Geometry check sheet. Reference: the model listing, model coordinates, mm. A direction names the side the tool comes from. Give positions to 0.01 mm unless a question says otherwise; leave off trailing zeros. Loops run counter-clockwise (first coordinate to the right, second up) from the corner with the lowest first, then second, coordinate; pieces in that order, holes last. Notation, with made-up numbers: (25.25, -20) - (58.25, -20) arc R16 ccw to (58.25, -16) - close; hole circle Ø7 at (-34.5, -17.5). An arc over 180 degrees is marked (long way). Write item = value, one per line. Start each with the question number.
from build123d import *

# Parameters (mm, degrees)
BOSS_EXTRUDE1_DEPTH = 2
SKETCH2_R           = 4
SKETCH2_R_2         = 3
BOSS_EXTRUDE2_DEPTH = 3.5
FILLET1_R           = 2.5
SKETCH3_R           = 1.5
CUT_EXTRUDE1_DEPTH  = 2


with BuildPart() as part:
    # Sketch1 → Boss-Extrude1 (new body)
    with BuildSketch(Plane(origin=(0, 0, 0), x_dir=(1, 0, 0), z_dir=(0, 1, 0))):
        with BuildLine():
            Line((-24.810790305, 12.959420841), (-17.699288905, 2.803144292))
            ThreePointArc((-17.699288905, 2.803144292), (-17.300062844, 1.904277974), (-17.699288905, 1.005411656))
            Line((-17.699288905, 1.005411656), (-24.810790305, -9.150864893))
            ThreePointArc((-24.810790305, -9.150864893), (-24.5530862, -12.096436293), (-21.6075148, -12.354140399))
            Line((-21.6075148, -12.354140399), (-11.45123825, -5.242638998))
            ThreePointArc((-11.45123825, -5.242638998), (-10.552371933, -4.843412937), (-9.653505615, -5.242638998))
            Line((-9.653505615, -5.242638998), (0.502770934, -12.354140399))
            ThreePointArc((0.502770934, -12.354140399), (3.448342335, -12.096436293), (3.70604644, -9.150864893))
            Line((3.70604644, -9.150864893), (-3.40545496, 1.005411656))
            ThreePointArc((-3.40545496, 1.005411656), (-3.804681022, 1.904277974), (-3.40545496, 2.803144292))
            Line((-3.40545496, 2.803144292), (3.70604644, 12.959420841))
            ThreePointArc((3.70604644, 12.959420841), (3.448342335, 15.904992242), (0.502770934, 16.162696347))
            Line((0.502770934, 16.162696347), (-9.653505615, 9.051194947))
            ThreePointArc((-9.653505615, 9.051194947), (-10.552371933, 8.651968885), (-11.45123825, 9.051194947))
            Line((-11.45123825, 9.051194947), (-21.6075148, 16.162696347))
            ThreePointArc((-21.6075148, 16.162696347), (-24.5530862, 15.904992242), (-24.810790305, 12.959420841))
        make_face()
    extrude(amount=BOSS_EXTRUDE1_DEPTH)

    # Sketch2 → Boss-Extrude2 (add)
    with BuildSketch(Plane.XZ):
        with Locations(Location((-10.552371933, -1.904277974, 0), (0, 0, 90))):
            Circle(SKETCH2_R)
        with Locations(Location((-10.552371933, -1.904277974, 0), (0, 0, 270))):
            Circle(SKETCH2_R_2, mode=Mode.SUBTRACT)
    extrude(amount=BOSS_EXTRUDE2_DEPTH)

    # Fillet1
    fillet1_edges = [part.edges().sort_by_distance(p)[0] for p in [
        (-10.552371933, 0, -5.904277974),
    ]]
    fillet(fillet1_edges, radius=FILLET1_R)

    # Sketch3 → Cut-Extrude1 (cut)
    with BuildSketch(Plane.XZ):
        with Locations(Location((-10.552371933, -1.904277974, 0), (0, 0, 270))):
            Circle(SKETCH3_R)
    extrude(amount=-CUT_EXTRUDE1_DEPTH, mode=Mode.SUBTRACT)


solid = part.part
1) Cross-section at C-C on y = 0.45. Enter the section's corners in (x, z).
2) Release check for a two-part mould opening along X. For faces 1 (the face through (-21.305, 0.986, -7.952)), 2 (the face through (-7.004, -2.993, -0.059)), 3 (the face through (0.1, 0.99, -7.81)), 4 (the face through (3.416, 0.986, 12.128)) record: pulls with the +X half, pulls with the -X half, needs draft (parallel to the pull), parting line crosses it, or undercut.
3) Cross-section at D-D on y = -1.6. Enter the section's corners in (x, z), and give its area (3 significant figures).
4) Material ranges on line 1 along Y through (x, z) = (-17.5, 0.5); line 2 along Z through (x, y) = (-22.5, 1.5); line 3 along Z through (x, y) = (-11.75, -0.9), recorded low to high.
5) Cross-section at A-A on x = -20.5. Enter the section's corners in (y, z), and give its area (3 significant figures).
6) Cross-section at B-B on z = -14.5. Enter the section's corners in (x, y), and give its area (3 significant figures).
7) Tool access check on faces 5 (the face through (-7.58, -1.73, -1.51)), 6 (the face through (0.2, 0.986, 4.144)), 7 (the face through (-16.6, 0.99, 8.85)), 8 (the face through (-21.205, 0.986, 4.002)), 9 (the face through (-16.46, 0.99, -12.56)). Record the directions out of +Z, -Z, +X, -X, +Y, -Y that give a thin tool (end or side, any length) a straight path to the whole face; none if there is none.
8) Gauge pin test, flat ends, axial feed: P1, Ø3, axis at y = 0, z = 6.5, coming from the -X side; P2, Ø5, axis at x = -10.55, z = -1.9, coming from the -Y side; P3, Ø1.5, axis at y = -3, z = -6, coming from the -X side. Record the tip position at first contact, or that the pin passes through.
Checked values:
q1.outline = (-24.81, -12.96) arc R2.3 ccw to (-21.61, -16.16) - (-11.45, -9.05) arc R1.21 cw to (-9.65, -9.05) - (0.5, -16.16) arc R2.3 ccw to (3.71, -12.96) - (-3.41, -2.8) arc R1.21 cw to (-3.41, -1.01) - (3.71, 9.15) arc R2.3 ccw to (0.5, 12.35) - (-9.65, 5.24) arc R1.21 cw to (-11.45, 5.24) - (-21.61, 12.35) arc R2.3 ccw to (-24.81, 9.15) - (-17.7, -1.01) arc R1.21 cw to (-17.7, -2.8) - close; hole circle Ø3 at (-10.55, -1.9)
q2.face_1 = pulls with the -X half
q2.face_2 = parting line crosses it
q2.face_3 = pulls with the +X half
q2.face_4 = undercut
q3.outline = circle Ø8.34 at (-10.55, -1.9); hole circle Ø6 at (-10.55, -1.9)
q3.area = 26.3 mm²
q4.line_1 = 0 to 2
q4.line_2 = -16.54 to -9.66, 5.85 to 12.73
q4.line_3 = -6.32 to -4.65, 0.85 to 2.52
q5.outline = (0, -15.39) - (2, -15.39) - (2, -6.8) - (0, -6.8) - close; (0, 2.99) - (2, 2.99) - (2, 11.58) - (0, 11.58) - close
q5.area = 34.3 mm²
q6.outline = (-25.22, 0) - (-19.23, 0) - (-19.23, 2) - (-25.22, 2) - close; (-1.87, 0) - (4.11, 0) - (4.11, 2) - (-1.87, 2) - close
q6.area = 23.9 mm²
q7.face_5 = -Y
q7.face_6 = +X, +Y, -Y
q7.face_7 = +Z, +Y, -Y
q7.face_8 = -X, +Y, -Y
q7.face_9 = -Z, +Y, -Y
q8.P1 = -24
q8.P2 = 0
q8.P3 = -12.74
